Geometry check sheet. Reference: the model listing, model coordinates, mm. Face numbers are marked on the shaded views. A direction names the side the tool comes from. Round coordinates to 2 decimals unless told otherwise and drop trailing zeros. Order: outer loops, then holes, each group sorted by start corner. A loop starts at its lowest first (then second) coordinate and runs counter-clockwise, first axis right, second up. Notation, with made-up numbers: (10, 32) - (22, 32) arc R22 ccw to (22, 67) - close; hole circle Ø6 at (40, 62.5). An arc over 180 degrees is marked (long way). Return JSON: item names as keys, results as strings. Group by question number.
Q1. Material ranges on line 1 along Y through (x, z) = (36.65, 37); line 2 along Y through (x, z) = (5, 37), recorded low to high.
Q2. Sectioned sample at B-B, the plane x = 21.15. Record the cut outline in (y, z), then the cut area to 3 significant figures.
Q3. Sectioned sample at C-C, the plane z = 8. Record the cut outline in (x, y).
Q4. Tool access check on the marked faces 1 and 2. Record the directions out of +Z, -Z, +X, -X, +Y, -Y that give a thin tool (end or side, any length) a straight path to the whole face; none if there is none.
Q5. Gauge pin test, flat ends, axial feed: pin 1 Ø3 at (x, y) = (36.65, 5.65) entering from +Z; pin 2 Ø3 at (y, z) = (22.5, 46.5) entering from -X. Record the tip position at first contact, or that the pin passes through.
Q6. Sectioned sample at A-A, the plane z = 37.5. Record the cut outline in (x, y).
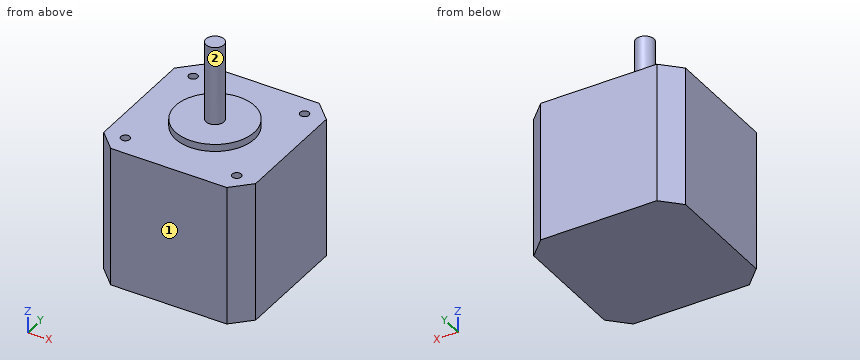
```python
from build123d import *

# Parameters (mm, degrees)
BOSS_EXTRUDE1_DEPTH       = 38.989
M3X0_5_TAPPED_HOLE1_D     = 2.5
M3X0_5_TAPPED_HOLE1_DEPTH = 5
M3X0_5_TAPPED_HOLE1_TIP   = 0.751075774
SKETCH4_R                 = 11
BOSS_EXTRUDE2_DEPTH       = 2
SKETCH5_R                 = 2.5
BOSS_EXTRUDE3_DEPTH       = 22


with BuildPart() as part:
    # Sketch1 → Boss-Extrude1 (new body)
    with BuildSketch(Plane.XY):
        Polygon((0, 37.3), (5, 42.3), (37.3, 42.3), (42.3, 37.3), (42.3, 5), (37.3, 0), (5, 0), (0, 5), align=None)
    extrude(amount=BOSS_EXTRUDE1_DEPTH)

    # M3x0.5 Tapped Hole1
    with Locations(Plane.XY.offset(38.989)):
        with Locations((5.65, 36.65), (36.65, 36.65), (36.65, 5.65), (5.65, 5.65)):
            Hole(M3X0_5_TAPPED_HOLE1_D / 2, depth=M3X0_5_TAPPED_HOLE1_DEPTH)
            with Locations((0, 0, -(M3X0_5_TAPPED_HOLE1_DEPTH + M3X0_5_TAPPED_HOLE1_TIP / 2))):  # 118° drill point
                Cone(0, M3X0_5_TAPPED_HOLE1_D / 2, M3X0_5_TAPPED_HOLE1_TIP, mode=Mode.SUBTRACT)

    # Sketch4 → Boss-Extrude2 (add)
    with BuildSketch(Plane.XY.offset(38.989)):
        with Locations(Location((21.15, 21.15, 0), (0, 0, 180))):
            Circle(SKETCH4_R)
    extrude(amount=BOSS_EXTRUDE2_DEPTH)

    # Sketch5 → Boss-Extrude3 (add)
    with BuildSketch(Plane.XY.offset(40.989)):
        with Locations((21.15, 21.15)):
            Circle(SKETCH5_R)
    extrude(amount=BOSS_EXTRUDE3_DEPTH)


solid = part.part
```
Reply:
{
 "1": {"line 1": "0 to 4.4, 6.9 to 35.4, 37.9 to 42.3", "line 2": "0 to 4.58, 6.72 to 35.58, 37.72 to 42.3"},
 "2": {"outline": "(0, 0) - (42.3, 0) - (42.3, 38.99) - (32.15, 38.99) - (32.15, 40.99) - (23.65, 40.99) - (23.65, 62.99) - (18.65, 62.99) - (18.65, 40.99) - (10.15, 40.99) - (10.15, 38.99) - (0, 38.99) - close", "area": "1,800 mm^2"},
 "3": {"outline": "(0, 5) - (5, 0) - (37.3, 0) - (42.3, 5) - (42.3, 37.3) - (37.3, 42.3) - (5, 42.3) - (0, 37.3) - close"},
 "4": {"face 1": "+Z, -Z, +X, -X, -Y", "face 2": "+Z"},
 "5": {"pin 1": "z = 38.99", "pin 2": "x = 18.65"},
 "6": {"outline": "(0, 5) - (5, 0) - (37.3, 0) - (42.3, 5) - (42.3, 37.3) - (37.3, 42.3) - (5, 42.3) - (0, 37.3) - close; hole circle Ø2.5 at (5.65, 5.65); hole circle Ø2.5 at (5.65, 36.65); hole circle Ø2.5 at (36.65, 5.65); hole circle Ø2.5 at (36.65, 36.65)"}
}
